Autodesk Inventor part; units mm, degrees
ref_plane "Lateral Sketch Plane" through (127, 1044.8596, 0) normal (0.5, 0.8660254, 0) x (-0.8660254, 0.5, 0)
ref_plane "YZ Plane" through (0, 0, 0) normal (1, 0, 0) x (0, 1, 0)
ref_plane "XZ Plane" through (0, 0, 0) normal (0, 1, 0) x (-1, 0, 0)
sketch "Sweep Sketch" plane through (0, 0, 0) normal (0, 0, 1) x (1, 0, 0)
  line L0 (-730.25, 0) -> (730.25, 0)
  line L1 (-476.25, 0) -> (127, 1044.8596)
  point P0 (0, 0)
  point P1 (0, 0)
  dimension "B_Dimension" = 1206.5
  dimension "C_Dimension" = 254
  dimension "A_Dimension" = 1206.5
  dimension "angle" = 60
sketch "Base Tube Profile Sketch" plane through (0, 0, 0) normal (1, 0, 0) x (0, 1, 0)
  circle A0 centre (0, 0) radius 304.8
  circle A1 centre (0, 0) radius 229.3874
  dimension "baseOD" = 609.6
  dimension "wallThickness" = 75.4126
sweep "Sweep1" add profiles "Base Tube Profile Sketch" path "Sweep Sketch" path curves L0
ref_plane "Lateral Sketch Plane" through (127, 1044.8596, 0) normal (0.5, 0.8660254, 0) x (-0.8660254, 0.5, 0)
sketch "Lateral Tube Profile Sketch" plane through (127, 1044.8596, 0) normal (0.5, 0.8660254, 0) x (-0.8660254, 0.5, 0)
  circle A0 centre (0, 0) radius 304.8
  circle A1 centre (0, 0) radius 229.3874
  point P0 (-412.4446, 0)
  dimension "lateralOD" = 609.6
  dimension "lateralWallThickness" = 75.4126
extrude "Extrusion1" add sketch "Lateral Tube Profile Sketch" against normal up to surface
extrude "Extrusion2" cut sketch "Lateral Tube Profile Sketch" against normal up to surface contours A1 surface through (0, 0, 0) normal (0, 1, 0)
equation "\"lateralOD\" = baseOD"
equation "\"lateralWallThickness\" = wallThickness"
equation "\"nominalSize\" = 609.6"
properties part number "LAT-S24-SCH160-60"
CAD build for the part. Positions are in the model's coordinates, mm. Give positions to 0.01 mm unless a question says otherwise; leave off trailing zeros. Write each loop counter-clockwise with the first axis right and the second up, starting at its lowest first coordinate (ties: lowest second). Pieces come first, ordered by that corner, then holes. Notation, with made-up numbers: (54.5, 15.5) - (105.5, 15.5) arc R19 cw to (105.5, 42.5) - close; hole circle Ø7 at (10.5, 18.5). An arc over 180 degrees is marked (long way). Put each result on its own line as item: value.
(1) Pull direction Z, two halves, no side cores. Call faces 1 (the cylindrical face through (10.224, -229.166, 10.086)), 2 (the flat face through (89.126, 1066.726, 227.2)), 3 (the cylindrical face through (-355.15, 791.2, 91.55)): released by +Z, released by -Z, zero draft, split by the parting line, or undercut.
Working result:
face 1: undercut
face 2: zero draft
face 3: split by the parting line
(2) Saw through at B-B (y = -149). List the corners of the cut face in (x, z).
Working result:
outline: (-730.25, -265.9) - (730.25, -265.9) - (730.25, -174.41) - (-730.25, -174.41) - close; (-730.25, 174.41) - (730.25, 174.41) - (730.25, 265.9) - (-730.25, 265.9) - close
(3) Wall check: L1, parallel to Y at x = 155, z = -58; L2, parallel to Z at x = 230, y = 0; L3, parallel to Y at x = 319, z = 166. Give the ranges that are in metal, low to high.
Working result:
L1: -299.23 to -221.93, 221.93 to 299.23, 494.9 to 649.49
L2: -304.8 to -229.39, 229.39 to 304.8
L3: -255.63 to -158.31, 158.31 to 255.63, 866.15 to 934.01
(4) Saw through at D-D (z = 261). List the corners of the cut face in (x, y), then the cut area to 3 significant figures.
Working result:
outline: (-730.25, -157.42) - (730.25, -157.42) - (730.25, 157.42) - (-203.59, 157.42) - (263.33, 966.15) - (-9.33, 1123.57) - (-567.14, 157.42) - (-730.25, 157.42) - close
area: 782,000 mm^2
(5) Saw through at A-A (z = 0). List the corners of the cut face in (x, y).
Working result:
outline: (-730.25, -304.8) - (730.25, -304.8) - (730.25, -229.39) - (-730.25, -229.39) - close; (-730.25, 229.39) - (-608.69, 229.39) - (-71.66, 1159.55) - (-136.96, 1197.26) - (-652.23, 304.8) - (-730.25, 304.8) - close; (-78.94, 229.39) - (730.25, 229.39) - (730.25, 304.8) - (51.68, 304.8) - (390.96, 892.46) - (325.66, 930.17) - close
(6) Saw through at C-C (x = 419.5). List the corners of the cut face in (y, z), then the cut area to 3 significant figures.
Working result:
outline: circle Ø609.6 at (0, 0); hole circle Ø458.77 at (0, 0)
area: 127,000 mm^2
(7) Drop flat-ended pins along their axis: pin 1 Ø1.5 at (y, z) = (365, 120.5) entering from +X; pin 2 Ø1 at (y, z) = (448.5, -210.5) entering from +X; pin 3 Ø8 at (y, z) = (718, 43) entering from +X. Give the stop position or say it passes through.
Working result:
pin 1: x = 58.33
pin 2: x = 37.85
pin 3: x = 289.12
